Geometry: final body of the model. Coordinates: model frame, mm. A direction names the side the tool comes from. Round coordinates to 2 decimals unless told otherwise and drop trailing zeros. Loops run counter-clockwise (first coordinate to the right, second up) from the corner with the lowest first, then second, coordinate; pieces in that order, holes last. Notation, with made-up numbers: (36.25, 77.25) - (91.25, 77.25) arc R19 ccw to (91.25, 100.25) - close; hole circle Ø10 at (73, 77.5). An arc over 180 degrees is marked (long way). Return JSON: item names as keys, results as strings. Group by question number.
1. Material intervals for probe 1 along Y at (x, z) = (-0.25, -21.5); probe 2 along Z at (x, y) = (-5.5, 1.5); probe 3 along Y at (x, z) = (1.5, -11), sorted ascending.
2. Section C-C on z = -18. Return loops of the section in (x, y).
3. Section A-A on y = 0. Return loops of the section in (x, z), and give its area (3 significant figures).
4. First-contact query: pin 1 Ø1.5 at (x, z) = (0.5, 6.5) entering from +Y; pin 2 Ø8 at (x, z) = (5.5, -2.5) entering from +Y; pin 3 Ø1.5 at (x, z) = (2.5, -12) entering from -Y. Flat tips, straight axial feed; report the tip coordinate or a pass-through.
5. Set-up query: faces 4 (the face through (-1.08, -4.88, 0.6)), 5 (the face through (0, 0, -25)). Return all of +Z, -Z, +X, -X, +Y, -Y with unobstructed straight access to the full face (end or side cutting, diameter ignored); none if empty.
6. Draft query along Z for faces 1 (the face through (0, 0, 27)), 2 (the face through (5.2, 0.1, 25)), 3 (the face through (-1.73, -7.81, 25.99)). Return one class per face: +Z half, -Z half, draft (parallel to the pull), parting line (faces both ways), or undercut.
7. Section D-D on x = -6. Return loops of the section in (y, z).
from build123d import *

# Parameters (mm, degrees)
SKETCH1_R           = 5
BOSS_EXTRUDE1_DEPTH = 25
FILLET3_R           = 0.5
BOSS_EXTRUDE2_START = 25
SKETCH2_R           = 8
BOSS_EXTRUDE2_DEPTH = 2


with BuildPart() as part:
    # Sketch1 → Boss-Extrude1 (new, symmetric)
    with BuildSketch(Plane.XY):
        Circle(SKETCH1_R)
    extrude(amount=BOSS_EXTRUDE1_DEPTH, both=True)

    # Fillet3
    fillet3_edges = [part.edges().sort_by_distance(p)[0] for p in [
        (-5, 0, -25),
    ]]
    fillet(fillet3_edges, radius=FILLET3_R)

    # Sketch2 → Boss-Extrude2 (add)
    with BuildSketch(Plane.XY.offset(BOSS_EXTRUDE2_START)):
        Circle(SKETCH2_R)
    extrude(amount=BOSS_EXTRUDE2_DEPTH)


solid = part.part
Taken from the geometry:
{
 "1": {"probe 1": "-4.99 to 4.99", "probe 2": "25 to 27", "probe 3": "-4.77 to 4.77"},
 "2": {"outline": "circle Ø10 at (0, 0)"},
 "3": {"outline": "(-8, 25) - (-5, 25) - (-5, -24.5) arc R0.5 ccw to (-4.5, -25) - (4.5, -25) arc R0.5 ccw to (5, -24.5) - (5, 25) - (8, 25) - (8, 27) - (-8, 27) - close", "area": "532 mm2"},
 "4": {"pin 1": "y = 5", "pin 2": "y = 4.77", "pin 3": "y = -4.68"},
 "5": {"face 4": "-Z", "face 5": "-Z, +X, -X, +Y, -Y"},
 "6": {"face 1": "+Z half", "face 2": "-Z half", "face 3": "draft"},
 "7": {"outline": "(-5.29, 25) - (5.29, 25) - (5.29, 27) - (-5.29, 27) - close"}
}
